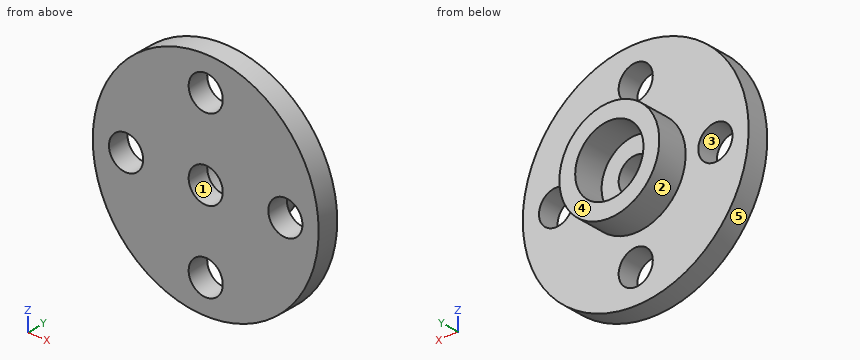
Autodesk Inventor part; units mm, degrees
ref_plane "YZ Plane" through (0, 0, 0) normal (1, 0, 0) x (0, 1, 0)
ref_plane "XZ Plane" through (0, 0, 0) normal (0, 1, 0) x (-1, 0, 0)
ref_plane "XY Plane" through (0, 0, 0) normal (0, 0, 1) x (1, 0, 0)
sketch "Sketch14" plane through (0, 0, 0) normal (0, 1, 0) x (-1, 0, 0)
  circle A0 centre (0, 0) radius 9.925
  circle A1 centre (0, 0) radius 7 construction
  circle A2 centre (7, 0) radius 1.5
  circle A3 centre (0, 7) radius 1.5
  circle A4 centre (-7, 0) radius 1.5
  circle A5 centre (0, -7) radius 1.5
  circle A6 centre (0, 0) radius 1.5
  dimension "d70" = 14
  dimension "d63" = 19.85
  dimension "d64" = 3
  dimension "d67" = 360
  dimension "d71" = 3
extrude "Extrusion11" add sketch "Sketch14" along normal blind 1.9
sketch "Sketch15" plane through (0, 1.9, 0) normal (0, 1, 0) x (1, 0, 0)
  circle A0 centre (0, 0) radius 1.5
  circle A1 centre (0, 0) radius 4.39
  circle A2 centre (0, 0) radius 3
  dimension "d74" = 8.78
  dimension "d75" = 6
extrude "Extrusion12" add sketch "Sketch15" along normal blind 2.7 contours A1
properties part number "ServoDrive" material "Steel"
Verification items for the finished model (mm, model axes). Face numbers are marked on the shaded views. A direction names the side the tool comes from. Coordinates: 2 decimals unless noted, no trailing zeros. Loops run counter-clockwise (first coordinate to the right, second up) from the corner with the lowest first, then second, coordinate; pieces in that order, holes last. Notation, with made-up numbers: (74, 68) - (110, 68) arc R21 cw to (110, 72) - close; hole circle Ø6 at (12.25, -18.75). An arc over 180 degrees is marked (long way). Return JSON: item names as keys, results as strings.
1. Section check B-B, the plane x = 0. Record the boundary of the cut face in (y, z) (3 decimals), then the cut area to 3 significant figures.
Established:
{"outline": "(0, -9.925) - (1.9, -9.925) - (1.9, -8.5) - (0, -8.5) - close; (0, -5.5) - (1.9, -5.5) - (1.9, -4.39) - (4.6, -4.39) - (4.6, -3) - (1.9, -3) - (1.9, -1.5) - (0, -1.5) - close; (0, 1.5) - (1.9, 1.5) - (1.9, 3) - (4.6, 3) - (4.6, 4.39) - (1.9, 4.39) - (1.9, 5.5) - (0, 5.5) - close; (0, 8.5) - (1.9, 8.5) - (1.9, 9.925) - (0, 9.925) - close", "area": "28.1 mm2"}
2. Section check A-A, the plane z = 0. Record the boundary of the cut face in (x, y) (3 decimals).
Established:
{"outline": "(-9.925, 0) - (-8.5, 0) - (-8.5, 1.9) - (-9.925, 1.9) - close; (-5.5, 0) - (-1.5, 0) - (-1.5, 1.9) - (-3, 1.9) - (-3, 4.6) - (-4.39, 4.6) - (-4.39, 1.9) - (-5.5, 1.9) - close; (1.5, 0) - (5.5, 0) - (5.5, 1.9) - (4.39, 1.9) - (4.39, 4.6) - (3, 4.6) - (3, 1.9) - (1.5, 1.9) - close; (8.5, 0) - (9.925, 0) - (9.925, 1.9) - (8.5, 1.9) - close"}
3. Thickness scan on L1, parallel to Z at x = 0, y = 1.05 (3 decimals); L2, parallel to X at y = 2.6, z = 0; L3, parallel to X at y = 1.7, z = -0.5. Record the ranges inside material, lowest first.
Established:
{"L1": "z = -9.925 to -8.5, -5.5 to -1.5, 1.5 to 5.5, 8.5 to 9.925", "L2": "x = -4.39 to -3, 3 to 4.39", "L3": "x = -9.91 to -8.41, -5.59 to -1.41, 1.41 to 5.59, 8.41 to 9.91"}
4. Go/stop test with flat-tipped pins: pin 1 (4 mm diameter, centred on x = 7, z = 0, fed in from +Y); pin 2 (2 mm diameter, centred on x = -2.5, y = 2, fed in from -Z). Record where each tip stops, or that it passes through.
Established:
{"pin 1": "stops at y = 1.9", "pin 2": "stops at z = -9.81"}
5. Section check C-C, the plane z = 7. Record the boundary of the cut face in (x, y), then the cut area to 3 significant figures.
Established:
{"outline": "(-7.04, 0) - (-1.5, 0) - (-1.5, 1.9) - (-7.04, 1.9) - close; (1.5, 0) - (7.04, 0) - (7.04, 1.9) - (1.5, 1.9) - close", "area": "21.0 mm2"}
6. Tool access check on the marked faces 1 and 2. Record the directions out of +Z, -Z, +X, -X, +Y, -Y that give a thin tool (end or side, any length) a straight path to the whole face; none if there is none.
Established:
{"face 1": "+Y, -Y", "face 2": "+Y"}
7. Mould release check, pull along X, two halves, no side actions. Record for the marked faces 3, 4 and 5: +X half, -X half, draft (parallel to the pull), parting line (faces both ways), or undercut.
Established:
{"face 3": "undercut", "face 4": "draft", "face 5": "parting line"}
8. Section check D-D, the plane y = 1.3. Record the boundary of the cut face in (x, z) (3 decimals).
Established:
{"outline": "circle Ø19.85 at (0, 0); hole circle Ø3 at (-7, 0); hole circle Ø3 at (0, -7); hole circle Ø3 at (0, 0); hole circle Ø3 at (0, 7); hole circle Ø3 at (7, 0)"}
